Geometry check sheet. Reference: the model listing, model coordinates, mm. Face numbers are marked on the shaded views. A direction names the side the tool comes from. Round coordinates to 2 decimals unless told otherwise and drop trailing zeros. Write each loop counter-clockwise with the first axis right and the second up, starting at its lowest first coordinate (ties: lowest second). Pieces come first, ordered by that corner, then holes. Notation, with made-up numbers: (17, 43.25) - (75, 43.25) arc R3 ccw to (75, 48.25) - close; hole circle Ø8 at (40.5, 14). An arc over 180 degrees is marked (long way). One line per question, with ' | ' between items. Start each with the question number.
from build123d import *

# Parameters (mm, degrees)
BOSS_EXTRUDE1_DEPTH = 25
SKETCH2_R           = 1.5
CUT_EXTRUDE1_DEPTH  = 26
SKETCH3_R           = 1.5
SKETCH3_W           = 25
SKETCH3_H           = 9
CUT_EXTRUDE2_DEPTH  = 10
SKETCH5_W           = 25
SKETCH5_H           = 1
CUT_EXTRUDE3_DEPTH  = 50


with BuildPart() as part:
    # Sketch1 → Boss-Extrude1 (new body)
    with BuildSketch(Plane.XY):
        Polygon((0, 27.931034483), (0, 12.931034483), (40, 12.931034483), (40, 7.931034483), (-5, 7.931034483), (-5, 27.931034483), align=None)
    extrude(amount=-BOSS_EXTRUDE1_DEPTH)

    # Sketch2 → Cut-Extrude1 (cut)
    with BuildSketch(Plane.ZY.offset(5)):
        with Locations((-22, 22.931034483)):
            Circle(SKETCH2_R)
        with Locations((-3, 22.931034483)):
            Circle(SKETCH2_R)
        with Locations((-3, 14.931034483)):
            Circle(SKETCH2_R)
        with Locations((-22, 14.931034483)):
            Circle(SKETCH2_R)
    extrude(amount=-CUT_EXTRUDE1_DEPTH, mode=Mode.SUBTRACT)

    # Sketch3 → Cut-Extrude2 (cut)
    with BuildSketch(Plane.XZ.offset(-7.931034483)):
        with Locations((6.802030066, -3.75)):
            Circle(SKETCH3_R)
        with Locations((6.802030066, -21.25)):
            Circle(SKETCH3_R)
        with Locations((27.5, -12.5)):
            Rectangle(SKETCH3_W, SKETCH3_H)
    extrude(amount=-CUT_EXTRUDE2_DEPTH, mode=Mode.SUBTRACT)

    # Sketch5 → Cut-Extrude3 (cut)
    with BuildSketch(Plane.XZ.offset(-7.931034483)):
        with Locations((27.5, -7.5)):
            Rectangle(SKETCH5_W, SKETCH5_H)
        with Locations((27.5, -17.5)):
            Rectangle(SKETCH5_W, SKETCH5_H)
    extrude(amount=-CUT_EXTRUDE3_DEPTH, mode=Mode.SUBTRACT)


solid = part.part
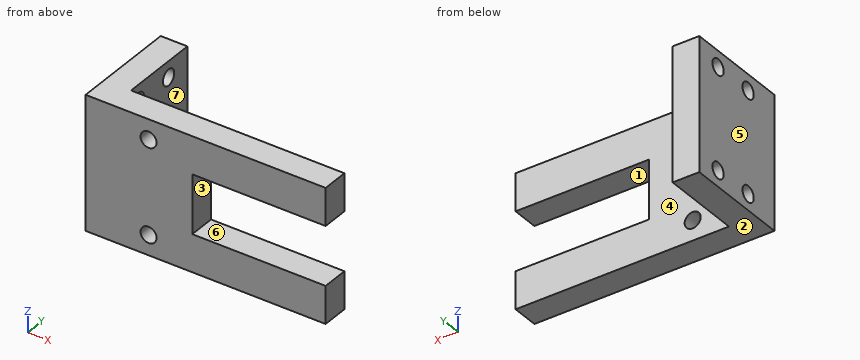
Q1. Section check B-B, the plane y = 10.25. Record the cut outline in (x, z).
Q2. Thickness scan on line 1 (Y direction, x = -3.6, z = -3); line 2 (Z direction, x = -0.5, y = 23); line 3 (X direction, y = 12.25, z = -15.5). Record the ranges inside material, lowest first.
Q3. Go/stop test with flat-tipped pins: P1, Ø12, axis at y = 19.5, z = -17, coming from the +X side; P2, Ø12.5, axis at x = 20.5, z = -14, coming from the +Y side; P3, Ø1.5, axis at y = 11.5, z = -11, coming from the +X side. Record where each tip stops, or that it passes through.
Q4. Section check D-D, the plane z = -5.75. Record the cut outline in (x, y), then the cut area to 3 significant figures.
Q5. Draft check along Z on the marked faces 1, 2, 3 and 4. Enter one of: pulls with the +Z half, pulls with the -Z half, needs draft (parallel to the pull), parting line crosses it, or undercut.
Q6. Section check A-A, the plane x = 18. Record the cut outline in (y, z), then the cut area to 3 significant figures.
Q7. Set-up check for the marked faces 5, 6 and 7: record each of +Z, -Z, +X, -X, +Y, -Y from which the full face is reachable in a straight line by a thin tool's end or side.
Q8. Section check C-C, the plane z = -21.25. Record the cut outline in (x, y).
Result sheet:
1) outline: (-5, -25) - (40, -25) - (40, -18) - (15, -18) - (15, -7) - (40, -7) - (40, 0) - (-5, 0) - close; hole circle Ø3 at (6.8, -21.25); hole circle Ø3 at (6.8, -3.75)
2) line 1: 7.93 to 13.43, 16.43 to 21.43, 24.43 to 27.93 | line 2: -25 to -23.5, -20.5 to -4.5, -1.5 to 0 | line 3: -5 to 15
3) P1: x = 0 | P2: y = 12.93 | P3: x = 15
4) outline: (-5, 7.93) - (40, 7.93) - (40, 12.93) - (0, 12.93) - (0, 27.93) - (-5, 27.93) - close | area: 300 mm²
5) face 1: undercut | face 2: pulls with the -Z half | face 3: undercut | face 4: needs draft
6) outline: (7.93, -25) - (12.93, -25) - (12.93, -18) - (7.93, -18) - close; (7.93, -7) - (12.93, -7) - (12.93, 0) - (7.93, 0) - close | area: 70.0 mm²
7) face 5: +Z, -Z, -X, +Y, -Y | face 6: +X, +Y, -Y | face 7: +Z, -Z, +X, +Y
8) outline: (-5, 7.93) - (5.3, 7.93) - (5.3, 12.93) - (0, 12.93) - (0, 13.63) - (-5, 13.63) - close; (-5, 16.23) - (0, 16.23) - (0, 21.63) - (-5, 21.63) - close; (-5, 24.23) - (0, 24.23) - (0, 27.93) - (-5, 27.93) - close; (8.3, 7.93) - (40, 7.93) - (40, 12.93) - (8.3, 12.93) - close
